Design review of the part shown in the three views and the two pictorial views. Dimensions are in mm from the part's minimum x, y and z. A direction names the side the tool comes from. Round coordinates to 2 decimals unless told otherwise and drop trailing zeros. Loops run counter-clockwise (first coordinate to the right, second up) from the corner with the lowest first, then second, coordinate; pieces in that order, holes last.
1. Clearance check with a flat-ended pin moving along its axis: pin 1 Ø1.8 at (x, z) = (6, 10) entering from +Y. State where the tip first meets the part, or that it passes through.
2. Tool access review of the marked faces 1 and 2: name each direction out of +Z, -Z, +X, -X, +Y, -Y from which nothing blocks a thin tool from reaching the whole face with its end or side.
3. Consider section D-D on x = 2. State the section outline as (y, z) points.
4. Consider section A-A on y = 0.8. State the section outline as (x, z) points, then the cut area to 3 significant figures.
5. To check wall thickness, follow line 1 along Z through (x, y) = (3.5, 3.5); line 2 along X through (y, z) = (0.65, 7.75); line 3 along X through (y, z) = (1.95, 7.5). State the ranges of each line that lie inside material, in increasing order.
6. Draft analysis for pull direction X (two halves, no side actions). For the marked faces 3, 4, 5 and 6, state which applies: released by +X, released by -X, zero draft, split by the parting line, or undercut.
7. Consider section C-C on z = 4.5. State the section outline as (x, y) points.
8. Consider section B-B on x = 3.7. State the section outline as (y, z) points, then the cut area to 3 significant figures.
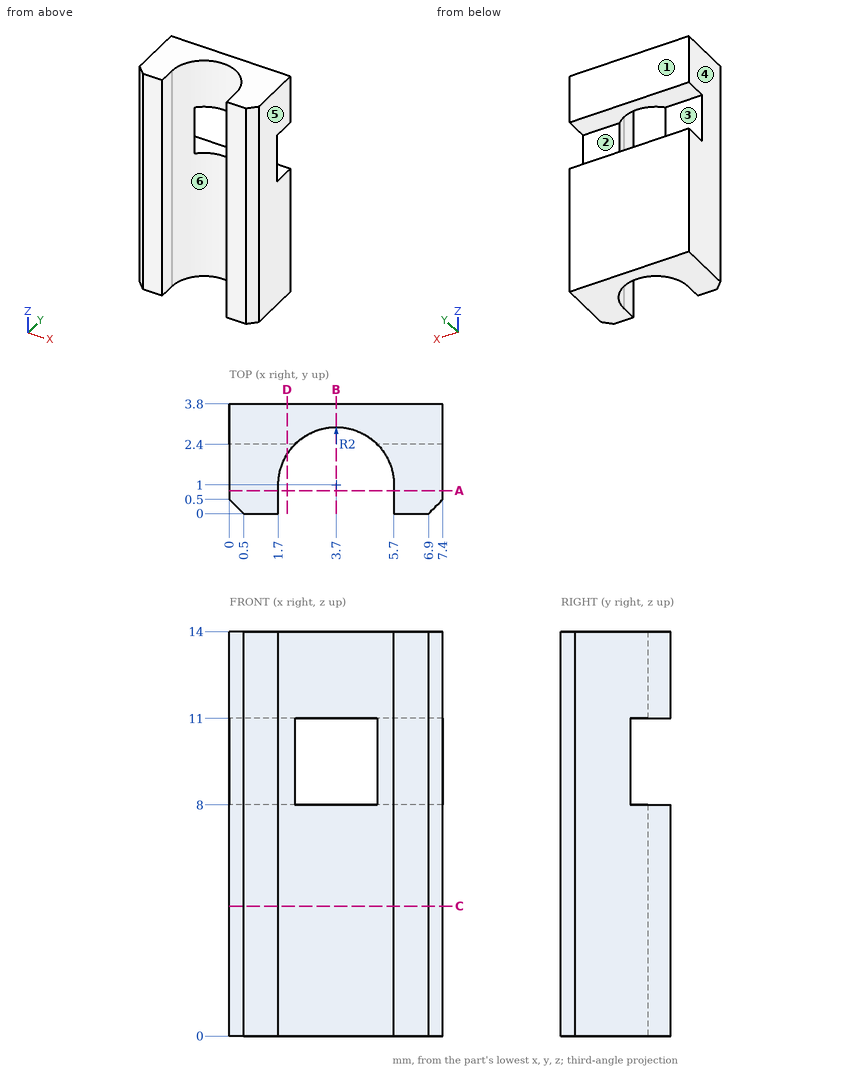
Resolved:
1. pin 1: stops at y = 2.4
2. face 1: +Z, -Z, +X, -X, +Y
2. face 2: +X, -X, +Y
3. outline: (2.05, 0) - (3.8, 0) - (3.8, 8) - (2.4, 8) - (2.4, 11) - (3.8, 11) - (3.8, 14) - (2.05, 14) - close
4. outline: (0, 0) - (1.7, 0) - (1.7, 14) - (0, 14) - close; (5.7, 0) - (7.4, 0) - (7.4, 14) - (5.7, 14) - close
4. area: 47.6 mm2
5. line 1: z = 0 to 8, 11 to 14
5. line 2: x = 0 to 1.7, 5.7 to 7.4
5. line 3: x = 0 to 1.94, 5.46 to 7.4
6. face 3: zero draft
6. face 4: released by -X
6. face 5: released by +X
6. face 6: undercut
7. outline: (0, 0.5) - (0.5, 0) - (1.7, 0) - (1.7, 1) arc R2 cw to (5.7, 1) - (5.7, 0) - (6.9, 0) - (7.4, 0.5) - (7.4, 3.8) - (0, 3.8) - close
8. outline: (3, 0) - (3.8, 0) - (3.8, 8) - (3, 8) - close; (3, 11) - (3.8, 11) - (3.8, 14) - (3, 14) - close
8. area: 8.80 mm2
